Here's the drawing with two shaded views (mm, measured from the low corner). I have some questions. A direction names the side the tool comes from. Round coordinates to 2 decimals unless told otherwise and drop trailing zeros. Write each loop counter-clockwise with the first axis right and the second up, starting at its lowest first coordinate (ties: lowest second). Pieces come first, ordered by that corner, then holes. Notation, with made-up numbers: M 9.25,59 L 45.25,59 A12 cw 45.25,76 Z; hole C 30.25,59.5 d1. An arc over 180 degrees is marked long. Use one line per item in the form item = value. Start each with the question number.
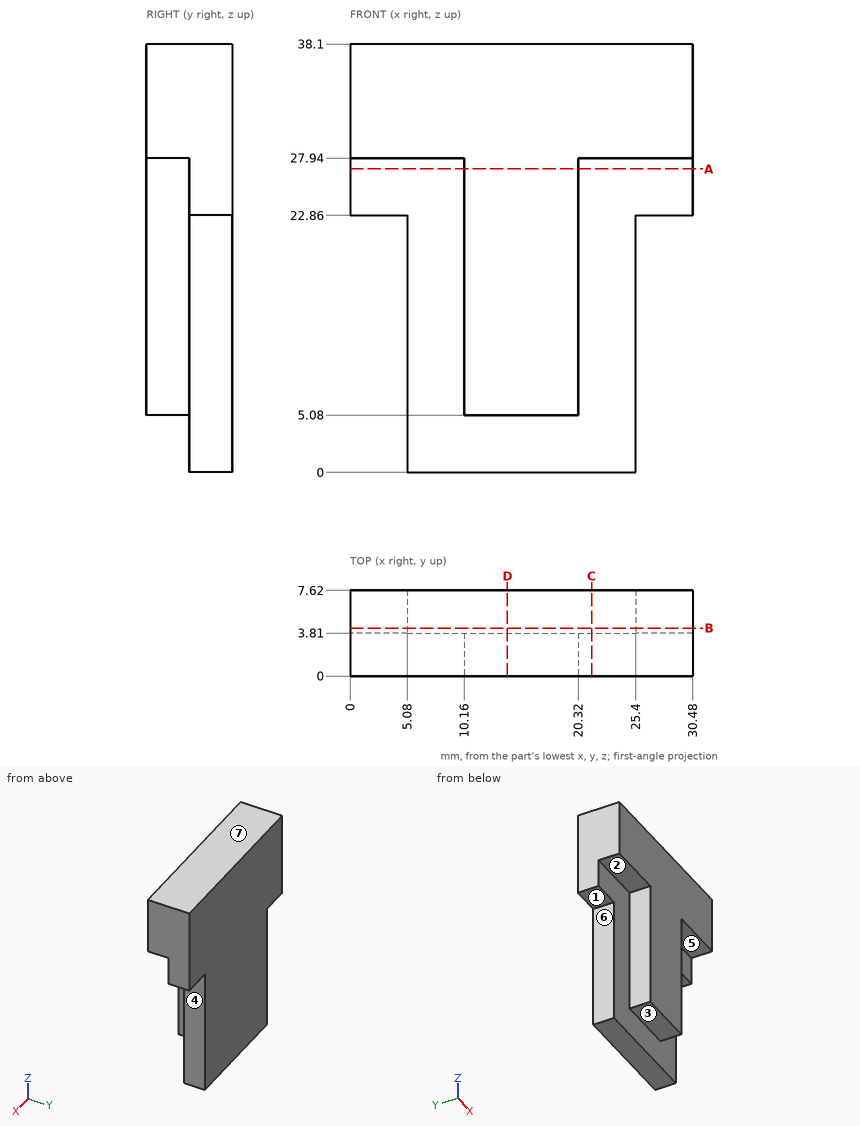
1. If we section it at D-D (x = 14): List the corners of the cut face in (y, z) for me.
2. If we section it at B-B (y = 4.25): List the corners of the cut face in (x, z) for me, and give its area (3 significant figures).
3. If we section it at C-C (x = 21.5): List the corners of the cut face in (y, z) for me, and give its area (3 significant figures).
4. If we mould it in two halves opening along Z, with no side actions, what happens to the marked faces 5, 6 and 7? For each: pulls with the +Z half, pulls with the -Z half, needs draft (parallel to the pull), parting line crosses it, or undercut.
5. If we section it at A-A (z = 27): List the corners of the cut face in (x, y) for me, and give its area (3 significant figures).
6. Please list where these lines run through material, in increasing order: line 1 along Y through (x, z) = (27, 27); line 2 along Z through (x, y) = (2, 4.75); line 3 along X through (y, z) = (7, 15).
7. Will these pins go through, and if not, where does the flat tip stop? pin 1 (1.5 mm diameter, centred on x = 4.5, y = 4.5, fed in from -Z); pin 2 (4 mm diameter, centred on y = 1, z = 12, fed in from -X); pin 3 (4 mm diameter, centred on x = 27.5, y = 6, fed in from -Z); pin 4 (1.1 mm diameter, centred on x = 5, y = 3, fed in from -Z).
8. Which directions (+Z, -Z, +X, -X, +Y, -Y) give clear straight access to the entire face, cutting with the end or side of a thin tool? Please do the marked faces 1, 2, 3 and 4.
Model answer:
q1.outline = M 0,5.08 L 3.81,5.08 L 3.81,0 L 7.62,0 L 7.62,38.1 L 0,38.1 Z
q2.outline = M 0,22.86 L 5.08,22.86 L 5.08,0 L 25.4,0 L 25.4,22.86 L 30.48,22.86 L 30.48,38.1 L 0,38.1 Z
q2.area = 929 mm2
q3.outline = M 0,27.94 L 3.81,27.94 L 3.81,0 L 7.62,0 L 7.62,38.1 L 0,38.1 Z
q3.area = 184 mm2
q4.face_5 = pulls with the -Z half
q4.face_6 = needs draft
q4.face_7 = pulls with the +Z half
q5.outline = M 0,3.81 L 10.16,3.81 L 10.16,0 L 20.32,0 L 20.32,3.81 L 30.48,3.81 L 30.48,7.62 L 0,7.62 Z
q5.area = 155 mm2
q6.line_1 = 3.81 to 7.62
q6.line_2 = 22.86 to 38.1
q6.line_3 = 5.08 to 25.4
q7.pin_1 = 0
q7.pin_2 = 10.16
q7.pin_3 = 22.86
q7.pin_4 = 27.94
q8.face_1 = -Z, -X, +Y, -Y
q8.face_2 = -Z, -X, -Y
q8.face_3 = -Z, +X, -X, -Y
q8.face_4 = -Z, +X, +Y, -Y
